Build history of the part. All positions in model axes, mm. Face numbers are marked on the shaded views. A direction names the side the tool comes from. Give positions to 0.01 mm unless a question says otherwise; leave off trailing zeros. Order: outer loops, then holes, each group sorted by start corner. A loop starts at its lowest first (then second) coordinate and runs counter-clockwise, first axis right, second up. Notation, with made-up numbers: (70, 18.5) -> (103, 18.5) arc R16 cw to (103, 39.5) -> close; hole circle Ø3 at (69, -38.5). An arc over 180 degrees is marked (long way). One line per item, written item: value. Start each with the question number.
(1) Pin check, flat tips, straight feed: pin 1 (1.5 mm diameter, centred on x = 1.5, y = 1.5, fed in from +Z); pin 2 (3 mm diameter, centred on x = -1, z = 5.5, fed in from -Y); pin 3 (1 mm diameter, centred on x = 1.5, z = 2.5, fed in from +Y). Stop position of each tip, or through.
(2) Which spindle directions (+Z, -Z, +X, -X, +Y, -Y) get a long thin tool onto all of the face, cutting with end or side? Do the marked faces 1 and 2. Say none if no direction does.
(3) Probe line 1 (Z direction, x = -0.05, y = -2.65); line 2 (Z direction, x = 0.8, y = 1.2); line 3 (X direction, y = 1.4, z = 3). List the from-to ranges inside material, lowest first.
(4) Saw through at A-A on x = 0. Give the cut face in (y, z), plus the area to 3 significant figures.
(5) Saw through at B-B on y = -1.6. Give the cut face in (x, z), plus the area to 3 significant figures.
(6) Saw through at C-C on z = 3.75. Give the cut face in (x, y).
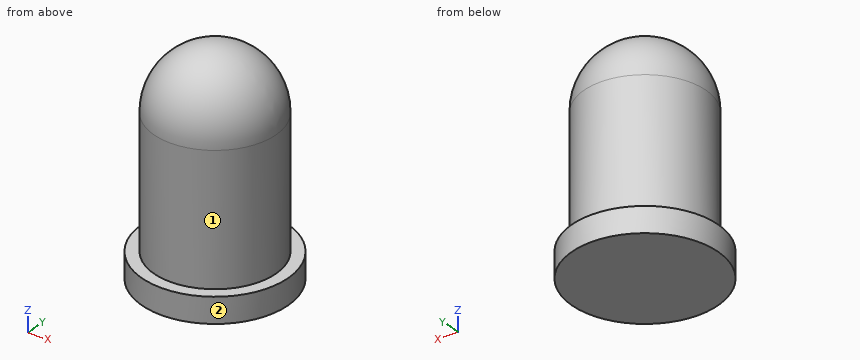
```python
from build123d import *

# Parameters (mm, degrees)
SKETCH1_R           = 2.5
BOSS_EXTRUDE1_DEPTH = 6.35
DOME1_FACE_RADIUS   = 2.5
DOME1_HEIGHT        = 2.54
SKETCH3_R           = 2.9972
BOSS_EXTRUDE2_DEPTH = 1.0414


with BuildPart() as part:
    # Sketch1 → Boss-Extrude1 (new body)
    with BuildSketch(Plane.XY):
        Circle(SKETCH1_R)
    extrude(amount=BOSS_EXTRUDE1_DEPTH)

    # Dome1: a dome of height H over a round flat face of radius A is a cap of a sphere of radius (A * A + H * H) / (2 * H)
    dome1_r = (DOME1_FACE_RADIUS * DOME1_FACE_RADIUS + DOME1_HEIGHT * DOME1_HEIGHT) / (2 * DOME1_HEIGHT)
    dome1_base = Plane((0, 0, 6.35), z_dir=(0, 0, 1))
    with Locations(dome1_base.offset(DOME1_HEIGHT - dome1_r)):
        dome1_ball = Sphere(dome1_r, mode=Mode.PRIVATE)
    add(split(dome1_ball, bisect_by=dome1_base, keep=Keep.TOP, mode=Mode.PRIVATE))

    # Sketch3 → Boss-Extrude2 (add)
    with BuildSketch(Plane(origin=(0, 0, 0), x_dir=(-1, 0, 0), z_dir=(0, 0, -1))):
        Circle(SKETCH3_R)
    extrude(amount=-BOSS_EXTRUDE2_DEPTH)


solid = part.part
```
Results below:
1. pin 1: stops at z = 8.48
1. pin 2: stops at y = -2.5
1. pin 3: stops at y = 2.29
2. face 1: +Z
2. face 2: +Z, -Z
3. line 1: z = 0 to 1.04
3. line 2: z = 0 to 8.43
3. line 3: x = -2.07 to 2.07
4. outline: (-3, 0) -> (3, 0) -> (3, 1.04) -> (2.5, 1.04) -> (2.5, 6.35) arc R2.5 ccw (long way) to (-2.5, 6.35) -> (-2.5, 1.04) -> (-3, 1.04) -> close
4. area: 42.8 mm²
5. outline: (-2.53, 0) -> (2.53, 0) -> (2.53, 1.04) -> (1.92, 1.04) -> (1.92, 6.35) arc R1.92 ccw (long way) to (-1.92, 6.35) -> (-1.92, 1.04) -> (-2.53, 1.04) -> close
5. area: 31.6 mm²
6. outline: circle Ø5 at (0, 0)
